Check sheet for the modelled part. Datum: model origin and axes. Units: mm. Coordinates: 2 decimals unless noted, no trailing zeros. Order: outer loops, then holes, each group sorted by start corner. A loop starts at its lowest first (then second) coordinate and runs counter-clockwise, first axis right, second up.
1. Cross-section at C-C (x = -317). Enter the section's corners in (y, z), then the cut area to 3 significant figures.
2. Cross-section at A-A (y = -25.4). Enter the section's corners in (x, z).
3. Thickness scan on line 1 (Z direction, x = -194, y = -8); line 2 (X direction, y = -4.5, z = 84); line 3 (Z direction, x = -505, y = -31). Record the ranges inside material, lowest first.
4. Cross-section at D-D (z = 41). Enter the section's corners in (x, y).
5. Cross-section at B-B (z = 107.95). Enter the section's corners in (x, y).
6. Gauge pin test, flat ends, axial feed: pin 1 Ø2 at (x, y) = (4.5, -31.5) entering from +Z; pin 2 Ø1 at (x, y) = (468.5, -29) entering from -Z. Record the tip position at first contact, or that the pin passes through.
```python
from build123d import *

# Parameters (mm, degrees)
F1_DEPTH = 50.8
F3_R     = 19.05
F4_DEPTH = 101.6


with BuildPart() as f1:
    # F0 (on Front) → F1 (new body)
    with BuildSketch(Plane.XZ):
        Polygon((0, 69.85), (0, 0), (330.2, 0), (479.993808, 69.85), (609.6, 69.85), (609.6, 139.7), (479.993808, 139.7), (330.2, 69.85), align=None)
    extrude(amount=F1_DEPTH)

    # F2: F1 across plane


with BuildPart() as f1_1:
    add(f1.part)
    add(f1.part.mirror(Plane.YZ))

    # F3 (on face) → F4 (join)
    with BuildSketch(Plane.YZ.offset(609.6)):
        with Locations((-25.4, 107.95)):
            Circle(F3_R)
    extrude(amount=F4_DEPTH)

    # F5: F1 across plane


with BuildPart() as f1_2:
    add(f1_1.part)
    add(f1_1.part.mirror(Plane.YZ))


solid = f1_2.part
```
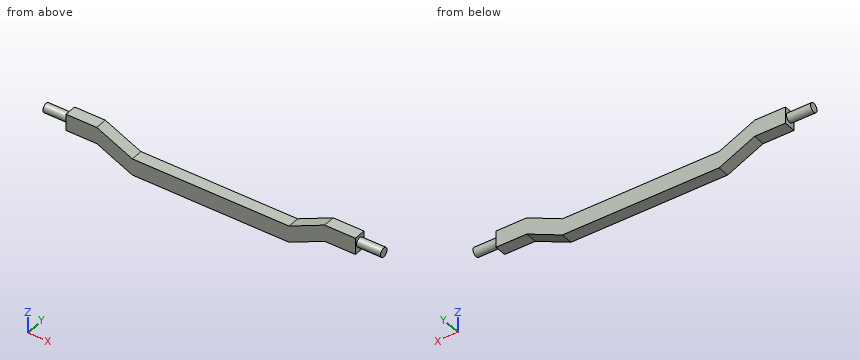
Data:
1. outline: (-50.8, 0) - (0, 0) - (0, 69.85) - (-50.8, 69.85) - close
1. area: 3,550 mm2
2. outline: (-711.2, 88.9) - (-609.6, 88.9) - (-609.6, 69.85) - (-479.99, 69.85) - (-330.2, 0) - (330.2, 0) - (479.99, 69.85) - (609.6, 69.85) - (609.6, 88.9) - (711.2, 88.9) - (711.2, 127) - (609.6, 127) - (609.6, 139.7) - (479.99, 139.7) - (330.2, 69.85) - (-330.2, 69.85) - (-479.99, 139.7) - (-609.6, 139.7) - (-609.6, 127) - (-711.2, 127) - close
3. line 1: z = 0 to 69.85
3. line 2: x = -609.6 to -360.54, 360.54 to 609.6
3. line 3: z = 69.85 to 139.7
4. outline: (-418.12, -50.8) - (418.12, -50.8) - (418.12, 0) - (-418.12, 0) - close
5. outline: (-711.2, -44.45) - (-609.6, -44.45) - (-609.6, -50.8) - (-411.91, -50.8) - (-411.91, 0) - (-609.6, 0) - (-609.6, -6.35) - (-711.2, -6.35) - close; (411.91, -50.8) - (609.6, -50.8) - (609.6, -44.45) - (711.2, -44.45) - (711.2, -6.35) - (609.6, -6.35) - (609.6, 0) - (411.91, 0) - close
6. pin 1: stops at z = 69.85
6. pin 2: stops at z = 64.26
